Build history of the part. All positions in model axes, mm. A direction names the side the tool comes from. Give positions to 0.01 mm unless a question says otherwise; leave off trailing zeros. Write each loop counter-clockwise with the first axis right and the second up, starting at its lowest first coordinate (ties: lowest second). Pieces come first, ordered by that corner, then holes.
from build123d import *

# Parameters (mm, degrees)
ESQUISSE1_W      = 29.5
ESQUISSE1_H      = 18.9
EXTRUSION1_DEPTH = 9.3
ESQUISSE2_W      = 29.5
ESQUISSE2_H      = 8.4
EXTRUSION2_DEPTH = 4.3
ESQUISSE3_W      = 7.2
ESQUISSE3_H      = 7.2
ESQUISSE3_R      = 3.25
ESQUISSE3_W_2    = 16.3
EXTRUSION3_DEPTH = 2
ESQUISSE4_R      = 2.5
EXTRUSION4_DEPTH = 2
CONG_1_R         = 2
ESQUISSE5_R      = 1.6
EXTRUSION5_DEPTH = 2
ESQUISSE6_W      = 10.1
ESQUISSE6_H      = 10.25
EXTRUSION6_DEPTH = 2
ESQUISSE7_W      = 10.1
ESQUISSE7_H      = 5
EXTRUSION7_DEPTH = 3


with BuildPart() as part:
    # Esquisse1 → Extrusion1 (new body)
    with BuildSketch(Plane(origin=(0, 0, 0), x_dir=(1, 0, 0), z_dir=(0, 1, 0))):
        with Locations((14.75, 9.45)):
            Rectangle(ESQUISSE1_W, ESQUISSE1_H)
    extrude(amount=EXTRUSION1_DEPTH)

    # Esquisse2 → Extrusion2 (add)
    with BuildSketch(Plane(origin=(0, 9.3, 0), x_dir=(1, 0, 0), z_dir=(0, 1, 0))):
        with Locations((14.75, 9.45)):
            Rectangle(ESQUISSE2_W, ESQUISSE2_H)
    extrude(amount=EXTRUSION2_DEPTH)

    # Esquisse3 → Extrusion3 (add)
    # profile 1 of 2: a face of its own
    with BuildSketch(Plane(origin=(0, 13.6, 0), x_dir=(1, 0, 0), z_dir=(0, 1, 0))):
        with Locations((4.5, 9.45)):
            Rectangle(ESQUISSE3_W, ESQUISSE3_H)
        with Locations(Location((4.5, 9.45, 0), (0, 0, 270))):
            Circle(ESQUISSE3_R, mode=Mode.SUBTRACT)
    # profile 2 of 2: a face of its own
    with BuildSketch(Plane(origin=(0, 13.6, 0), x_dir=(1, 0, 0), z_dir=(0, 1, 0))):
        with Locations((20.4, 9.45)):
            Rectangle(ESQUISSE3_W_2, ESQUISSE3_H)
        with Locations(Location((24.5, 9.45, 0), (0, 0, 270))):
            Circle(ESQUISSE3_R, mode=Mode.SUBTRACT)
    extrude(amount=EXTRUSION3_DEPTH)

    # Esquisse4 → Extrusion4 (add)
    with BuildSketch(Plane(origin=(0, 13.6, 0), x_dir=(1, 0, 0), z_dir=(0, 1, 0))):
        with Locations(Location((4.5, 9.45, 0), (0, 0, 90))):
            Circle(ESQUISSE4_R)
        with Locations(Location((24.5, 9.45, 0), (0, 0, 90))):
            Circle(ESQUISSE4_R)
    extrude(amount=EXTRUSION4_DEPTH)

    # Congé1
    cong_1_edges = [part.edges().sort_by_distance(p)[0] for p in [
        (4.5, 15.6, -6.95),
        (24.5, 15.6, -6.95),
    ]]
    fillet(cong_1_edges, radius=CONG_1_R - 0.0001)  # a hair under: the kernel refuses the full size

    # Esquisse5 → Extrusion5 (add)
    # profile 1 of 2: a face of its own
    with BuildSketch(Plane.XZ):
        with BuildLine():
            Line((0, -5.7), (-3.75, -5.7))
            ThreePointArc((-3.75, -5.7), (-7.5, -9.45), (-3.75, -13.2))
            Line((-3.75, -13.2), (0, -13.2))
            Line((0, -13.2), (0, -5.7))
        make_face()
        with Locations(Location((-3.75, -9.45, 0), (0, 0, 270))):
            Circle(ESQUISSE5_R, mode=Mode.SUBTRACT)
    # profile 2 of 2: a face of its own
    with BuildSketch(Plane.XZ):
        with BuildLine():
            Line((29.5, -5.7), (33.25, -5.7))
            ThreePointArc((33.25, -5.7), (37, -9.45), (33.25, -13.2))
            Line((33.25, -13.2), (29.5, -13.2))
            Line((29.5, -13.2), (29.5, -5.7))
        make_face()
        with Locations(Location((33.25, -9.45, 0), (0, 0, 90))):
            Circle(ESQUISSE5_R, mode=Mode.SUBTRACT)
    extrude(amount=-EXTRUSION5_DEPTH)

    # Esquisse6 → Extrusion6 (add)
    with BuildSketch(Plane(origin=(0, 9.3, 0), x_dir=(1, 0, 0), z_dir=(0, 1, 0))):
        with Locations((14.75, 0.125)):
            Rectangle(ESQUISSE6_W, ESQUISSE6_H)
    extrude(amount=EXTRUSION6_DEPTH)

    # Esquisse7 → Extrusion7 (add)
    with BuildSketch(Plane.XZ.offset(-9.3)):
        with Locations((14.75, 2.5)):
            Rectangle(ESQUISSE7_W, ESQUISSE7_H)
    extrude(amount=EXTRUSION7_DEPTH)


solid = part.part
1. 3-axis set-ups, long thin cutter, end or side, ignore diameter. For faces 1 (the face through (0.9, 15, -9)), 2 (the face through (-2, 1, -13.2)), 3 (the face through (15, 9.3, -16)): which of +Z, -Z, +X, -X, +Y, -Y reach the whole face in a straight line?
2. Saw through at D-D on z = -10.5. Count the separate pieces of the cut face and the enclosed holes in it, plus the area to 3 significant figures.
3. Mould opens along Z. For faces 4 (the face through (-2, 1, -5.7)), 5 (the face through (34.67, 0.99, -8.71)), 6 (the face through (25, 9.3, -3)) say: pulls with the +Z half, pulls with the -Z half, needs draft (parallel to the pull), parting line crosses it, or undercut.
4. Drill centre lines: line 1 along Z through (x, y) = (33.25, 0.85); line 2 along X through (y, z) = (15.1, -9.45); line 3 along Z through (x, y) = (15, 14.25). Where is each one in solid material? Low to high.
5. Drop flat-ended pins along their axis: pin 1 (1 mm diameter, centred on x = 6, y = 14.5, fed in from -Z); pin 2 (5 mm diameter, centred on x = 8.5, z = -10.5, fed in from -Y); pin 3 (8 mm diameter, centred on y = 7.5, z = -10.5, fed in from -X); pin 4 (2 mm diameter, centred on x = -5, z = -10, fed in from +Y). Give the stop position or say it passes through.
6. Saw through at A-A on x = 32.5. Give the cut face in (y, z).
7. Saw through at B-B on z = -2. Give the cut face in (x, y).
8. Saw through at C-C on y = 10. Give the cut face in (x, z), plus the area to 3 significant figures.
Outcome:
1. face 1: +Z, -Z, -X, +Y
1. face 2: -Z, -X, +Y, -Y
1. face 3: -Z, +X, -X, +Y
2. separate pieces: 3
2. enclosed holes: 0
2. area: 457 mm2
3. face 4: pulls with the +Z half
3. face 5: undercut
3. face 6: needs draft
4. line 1: z = -13.2 to -11.05, -7.85 to -5.7
4. line 2: x = 0.9 to 1.25, 2.68 to 6.32, 7.75 to 8.1, 12.25 to 21.25, 22.68 to 26.32, 27.75 to 28.55
4. line 3: z = -13.05 to -5.85
5. pin 1: stops at z = -13.05
5. pin 2: stops at y = 0
5. pin 3: stops at x = 0
5. pin 4: stops at y = 2
6. outline: (0, -13.2) - (2, -13.2) - (2, -10.86) - (0, -10.86) - close; (0, -8.04) - (2, -8.04) - (2, -5.7) - (0, -5.7) - close
7. outline: (0, 0) - (29.5, 0) - (29.5, 9.3) - (19.8, 9.3) - (19.8, 11.3) - (9.7, 11.3) - (9.7, 9.3) - (0, 9.3) - close
8. outline: (0, -13.65) - (29.5, -13.65) - (29.5, -5.25) - (19.8, -5.25) - (19.8, 5) - (9.7, 5) - (9.7, -5.25) - (0, -5.25) - close
8. area: 351 mm2
